Source: CAD feature listing. Evaluate the final solid. Frame: model axes, mm. Round coordinates to 2 decimals unless told otherwise and drop trailing zeros. Write each loop counter-clockwise with the first axis right and the second up, starting at its lowest first coordinate (ties: lowest second). Pieces come first, ordered by that corner, then holes. Notation, with made-up numbers: M 80,72 L 119,72 A19 cw 119,89 Z; hole C 79,-25.75 d11. An arc over 180 degrees is marked long. Use a Markdown table: item, result.
```python
from build123d import *

# Parameters (mm, degrees)
SKETCH1_R           = 52.832
SKETCH1_R_2         = 50.8
BOSS_EXTRUDE1_DEPTH = 457.2
CIRPATTERN1_COUNT   = 4
CIRPATTERN2_COUNT   = 8


with BuildPart() as part:
    # Sketch1 → Boss-Extrude1 (new body)
    with BuildSketch(Plane(origin=(0, 0, 0), x_dir=(1, 0, 0), z_dir=(0, 1, 0))):
        with Locations(Location((0, 0, 0), (0, 0, 270))):
            Circle(SKETCH1_R)
        with Locations(Location((0, 0, 0), (0, 0, 270))):
            Circle(SKETCH1_R_2, mode=Mode.SUBTRACT)
    extrude(amount=BOSS_EXTRUDE1_DEPTH)

    # Sketch4 → #2 Clearance Hole1 (revolve, cut)
    with BuildSketch(Plane(origin=(0, 96.9772, 52.832), x_dir=(0, -1, 0), z_dir=(1, 0, 0))):
        Polygon((0, 0), (0, 55.596569267), (1.2192, 54.864), (1.2192, 0), align=None)
    f_2_clearance_hole1 = revolve(axis=Axis((0, 96.9772, 59.182), (0, 0, -1)), mode=Mode.SUBTRACT)

    # Sketch6 → #8 Clearance Hole1 (revolve, cut)
    with BuildSketch(Plane(origin=(20.217931099, 406.4, 48.810403462), x_dir=(0.9238795325112864, 0, -0.38268343236509056), z_dir=(0, 1, 0))):
        Polygon((0, 0), (0, 56.214674586), (2.2479, 54.864), (2.2479, 0), align=None)
    f_8_clearance_hole1 = revolve(axis=Axis((22.647970894, 406.4, 54.677038493), (-0.38268343236509056, 0, -0.9238795325112865)), mode=Mode.SUBTRACT)

    # CirPattern1: #2 Clearance Hole1 ×4 about axis
    cirpattern1_axis = Axis((0, 457.2, 0), (0, -1, 0))
    for i in range(1, CIRPATTERN1_COUNT):
        add(f_2_clearance_hole1.rotate(cirpattern1_axis, i * 360 / CIRPATTERN1_COUNT), mode=Mode.SUBTRACT)

    # CirPattern2: #8 Clearance Hole1 ×8 about axis
    cirpattern2_axis = Axis((0, 457.2, 0), (0, -1, 0))
    for i in range(1, CIRPATTERN2_COUNT):
        add(f_8_clearance_hole1.rotate(cirpattern2_axis, i * 360 / CIRPATTERN2_COUNT), mode=Mode.SUBTRACT)


solid = part.part
```
Q1. Section B-B on z = 7. Return loops of the section in (x, y), plus the area to 3 significant figures.
Results are:
| item | result |
|---|---|
| outline | M -52.37,0 L -50.32,0 L -50.32,457.2 L -52.37,457.2 Z; M 50.32,0 L 52.37,0 L 52.37,457.2 L 50.32,457.2 Z |
| area | 1,880 mm^2 |
Q2. Mould query, pull axis Z, two halves, no side actions, for faces 1 (the cylindrical face through (15.87, 225.4, 50.39)), 2 (the cylindrical face through (-30.911, 225.4, -40.313)), 3 (the flat face through (43, 0, -28)). Classes: +Z half, -Z half, draft (parallel to the pull), parting line (faces both ways), or undercut.
Results are:
| item | result |
|---|---|
| face 1 | parting line |
| face 2 | undercut |
| face 3 | draft |
Q3. Line query: L1, parallel to Y at x = 0, z = 51.85; L2, parallel to Z at x = 0, y = 306; L3, parallel to X at y = 110.5, z = -3. Output: solid intervals per line, ascending.
Results are:
| item | result |
|---|---|
| L1 | 0 to 95.76, 98.2 to 457.2 |
| L2 | -52.83 to -50.8, 50.8 to 52.83 |
| L3 | -52.75 to -50.71, 50.71 to 52.75 |
Q4. Section C-C on y = 299.5. Return loops of the section in (x, z).
Results are:
| item | result |
|---|---|
| outline | C 0,0 d105.66; hole C 0,0 d101.6 |
Q5. Section A-A on x = -6. Return loops of the section in (y, z), plus the area to 3 significant figures.
Results are:
| item | result |
|---|---|
| outline | M 0,-52.49 L 457.2,-52.49 L 457.2,-50.44 L 0,-50.44 Z; M 0,50.44 L 457.2,50.44 L 457.2,52.49 L 0,52.49 Z |
| area | 1,870 mm^2 |
Q6. First-contact query: pin 1 Ø1 at (y, z) = (386.5, -1) entering from -X; pin 2 Ø1.5 at (y, z) = (378.5, 38) entering from -X; pin 3 Ø1.5 at (y, z) = (96.98, 0) entering from +X; pin 4 Ø1 at (y, z) = (275, 20) entering from -X. Flat tips, straight axial feed; report the tip coordinate or a pass-through.
Results are:
| item | result |
|---|---|
| pin 1 | x = -52.83 |
| pin 2 | x = -37.47 |
| pin 3 | through |
| pin 4 | x = -49.1 |
